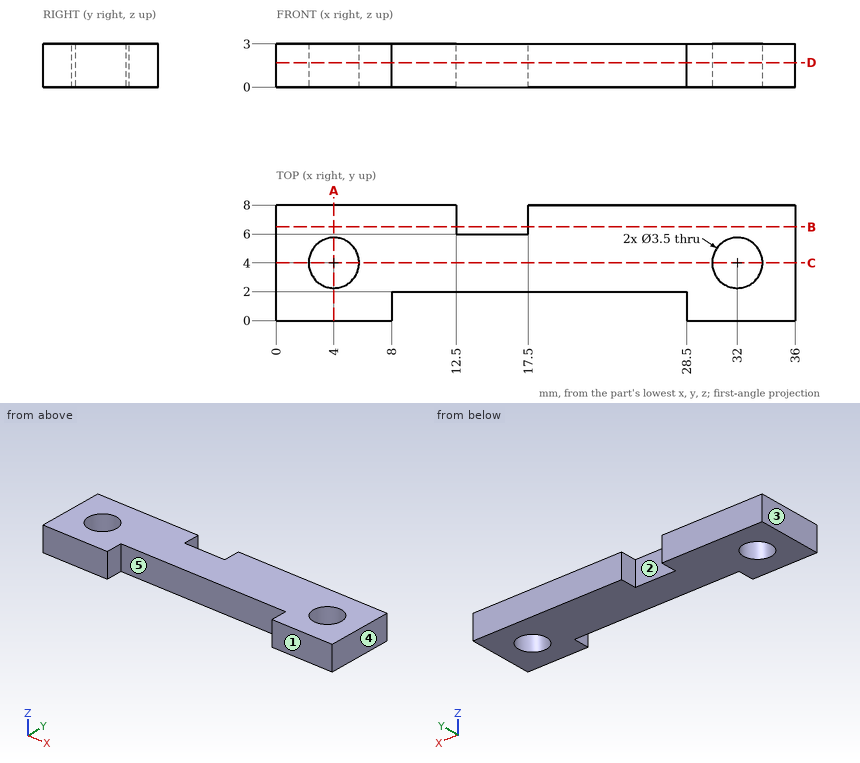
Geometry check sheet. Reference: drawing and pictorial views, mm from the part's lowest x, y, z. A direction names the side the tool comes from. Round coordinates to 2 decimals unless told otherwise and drop trailing zeros. Loops run counter-clockwise (first coordinate to the right, second up) from the corner with the lowest first, then second, coordinate; pieces in that order, holes last. Notation, with made-up numbers: (47.5, 15.25) - (66.5, 15.25) arc R31 cw to (66.5, 49.25) - close; hole circle Ø6 at (10.25, 81). An arc over 180 degrees is marked (long way). Use a Markdown table: item, result. Add a question column.
1. Section check D-D, the plane z = 1.7. Record the boundary of the cut face in (x, y), plus the area to 3 significant figures.
2. Gauge pin test, flat end, axial feed: pin 1 (0.9 mm diameter, centred on x = 18, z = 1, fed in from -Y). Record the tip position at first contact, or that the pin passes through.
3. Thickness scan on probe 1 along Y at (x, z) = (4, 1.6); probe 2 along X at (y, z) = (7.5, 1.6); probe 3 along X at (y, z) = (0.5, 2.1). Record the ranges inside material, lowest first. Write a range as [from, to].
4. Release check for a two-part mould opening along X. For the marked faces 3, 4 and 5 record: released by +X, released by -X, zero draft, split by the parting line, or undercut.
5. Section check C-C, the plane y = 4. Record the boundary of the cut face in (x, z).
6. Access from +Z, -Z, +X, -X, +Y, -Y to the whole of each face (thin tool, end or side, straight path). Record for the marked faces 1 and 2.
7. Section check A-A, the plane x = 4. Record the boundary of the cut face in (y, z).
8. Section check B-B, the plane y = 6.5. Record the boundary of the cut face in (x, z), plus the area to 3 significant figures.
Checks:
| question | item | result |
|---|---|---|
| 1 | outline | (0, 0) - (8, 0) - (8, 2) - (28.5, 2) - (28.5, 0) - (36, 0) - (36, 8) - (17.5, 8) - (17.5, 6) - (12.5, 6) - (12.5, 8) - (0, 8) - close; hole circle Ø3.5 at (4, 4); hole circle Ø3.5 at (32, 4) |
| 1 | area | 218 mm^2 |
| 2 | pin 1 | stops at y = 2 |
| 3 | probe 1 | y = [0, 2.25], [5.75, 8] |
| 3 | probe 2 | x = [0, 12.5], [17.5, 36] |
| 3 | probe 3 | x = [0, 8], [28.5, 36] |
| 4 | face 3 | released by -X |
| 4 | face 4 | released by +X |
| 4 | face 5 | undercut |
| 5 | outline | (0, 0) - (2.25, 0) - (2.25, 3) - (0, 3) - close; (5.75, 0) - (30.25, 0) - (30.25, 3) - (5.75, 3) - close; (33.75, 0) - (36, 0) - (36, 3) - (33.75, 3) - close |
| 6 | face 1 | +Z, -Z, +X, -X, -Y |
| 6 | face 2 | +Z, -Z, +Y |
| 7 | outline | (0, 0) - (2.25, 0) - (2.25, 3) - (0, 3) - close; (5.75, 0) - (8, 0) - (8, 3) - (5.75, 3) - close |
| 8 | outline | (0, 0) - (12.5, 0) - (12.5, 3) - (0, 3) - close; (17.5, 0) - (36, 0) - (36, 3) - (17.5, 3) - close |
| 8 | area | 93.0 mm^2 |
